Study the drawing (mm; zero at the part's minimum x, y, z) and answer. A direction names the side the tool comes from. Round coordinates to 2 decimals unless told otherwise and drop trailing zeros. Write each loop counter-clockwise with the first axis right and the second up, starting at its lowest first coordinate (ties: lowest second). Pieces come first, ordered by that corner, then holes. Notation, with made-up numbers: (2.25, 37) - (40.25, 37) arc R17 cw to (40.25, 48) - close; hole circle Ø5 at (-16, -36). An arc over 180 degrees is marked (long way). Use one line per item in the form item = value. Start each with the question number.
1) For the marked faces 1, 2 and 3, determine the directions among +Z, -Z, +X, -X, +Y, -Y from which every point of the face is accessible in a straight line to the end or side of a thin tool.
2) The part is cut by section C-C, the plane x = 11.5. Give the vertices of the cut face in (y, z).
3) The part is cut by section A-A, the plane z = 24. Give the vertices of the cut face in (x, y) (1 decimal).
4) The part is cut by section D-D, the plane z = 30. Give the vertices of the cut face in (x, y) (1 decimal), plus the area to 3 significant figures.
5) The part is cut by section B-B, the plane y = 6. Give the vertices of the cut face in (x, z), plus the area to 3 significant figures.
6) Consider line 1 along Z through (x, y) = (38.5, 36); line 2 along X through (y, z) = (7.5, 39.5); line 3 along Y through (x, z) = (19, 14). Determine where each line is inside the solid, lowest interval first. Write a range as from..to.
7) Each of these flat-tipped pins is pushed along its axis until it touches: pin 1 (4 mm diameter, centred on x = 33, y = 35, fed in from +Z); pin 2 (6 mm diameter, centred on y = 7.5, z = 34, fed in from +X); pin 3 (10 mm diameter, centred on x = 19, z = 25, fed in from +Y). Where does it stop, or does it pass through?
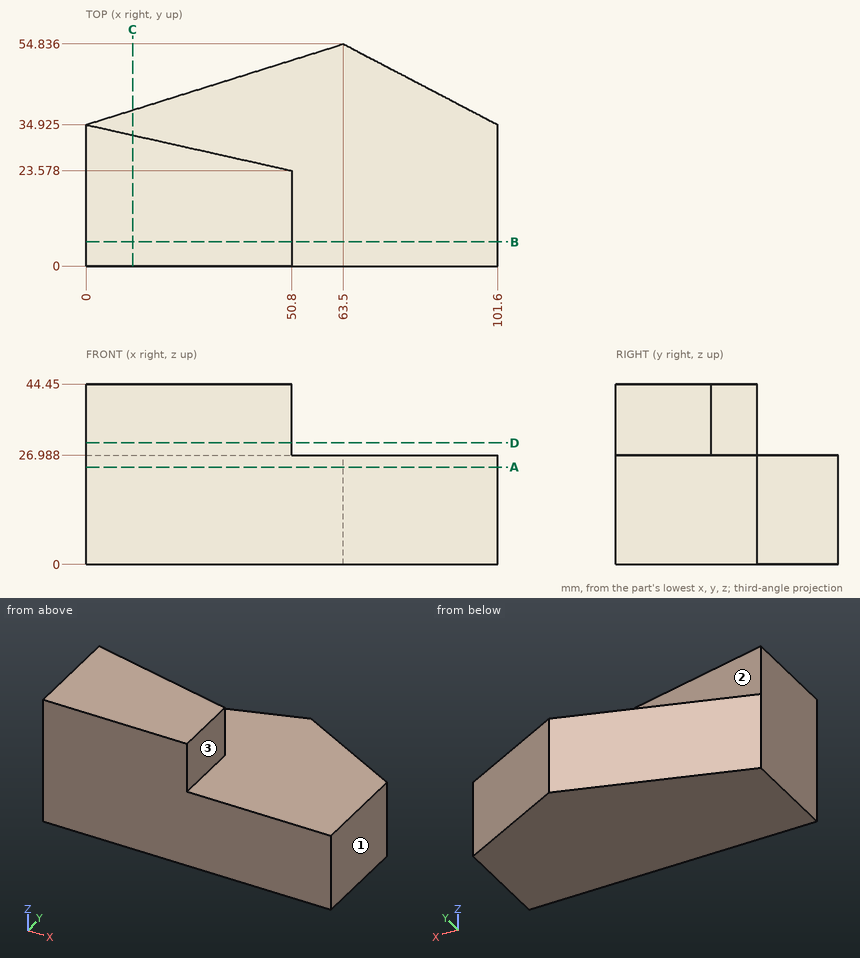
Geometry results:
q1.face_1 = +Z, -Z, +X, +Y, -Y
q1.face_2 = +Z, +X, +Y
q1.face_3 = +Z, +X, +Y, -Y
q2.outline = (0, 0) - (38.53, 0) - (38.53, 26.99) - (32.36, 26.99) - (32.36, 44.45) - (0, 44.45) - close
q3.outline = (0, 0) - (101.6, 0) - (101.6, 34.9) - (63.5, 54.8) - (0, 34.9) - close
q4.outline = (0, 0) - (50.8, 0) - (50.8, 23.6) - (0, 34.9) - close
q4.area = 1,490 mm2
q5.outline = (0, 0) - (101.6, 0) - (101.6, 26.99) - (50.8, 26.99) - (50.8, 44.45) - (0, 44.45) - close
q5.area = 3,630 mm2
q6.line_1 = 0..26.99
q6.line_2 = 0..50.8
q6.line_3 = 0..40.88
q7.pin_1 = 26.99
q7.pin_2 = 50.8
q7.pin_3 = 42.45
